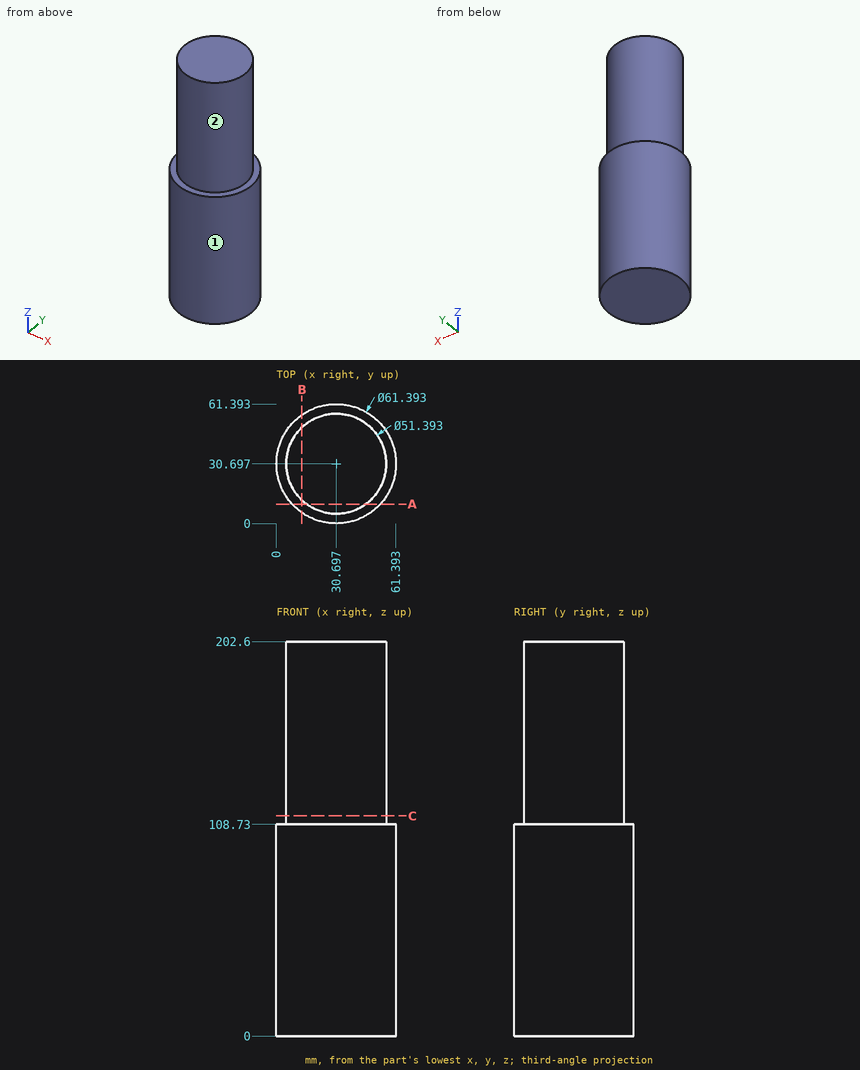
Could you check a few things on this drawing? It's one solid part, dimensions in mm from its lowest x, y, z. A direction names the side the tool comes from. Coordinates: 2 decimals unless noted, no trailing zeros. Loops run counter-clockwise (first coordinate to the right, second up) from the corner with the lowest first, then second, coordinate; pieces in that order, holes last. Notation, with made-up numbers: (28, -2) - (87, -2) arc R14 ccw to (87, 17) - close; hole circle Ø11 at (24.5, 18). An arc over 180 degrees is marked (long way). Answer as a JSON object with one key per item and string values. Group by question number.
Item 1: On a 3-axis mill with a long thin cutter (end or side, diameter ignored), from which of +Z, -Z, +X, -X, +Y, -Y can I reach the whole of each face in a straight line? I mean the marked faces 1 and 2. Say none if no direction works.
Item 2: If we section it at A-A (y = 10): List the corners of the cut face in (x, z) for me, plus the area to 3 significant figures.
Item 3: For pin 1 (1.5 mm diameter, centred on y = 27.5, z = 157.5, fed in from +X); pin 2 (5 mm diameter, centred on x = 29, z = 58, fed in from -Y); pin 3 (10 mm diameter, centred on x = 7, z = 135.5, fed in from -Y), each with a flat end and sliding along its axis, tell me the tip position at first contact or that it passes through.
Item 4: If I drill on L1, parallel to Z at x = 14, y = 55; L2, parallel to X at y = 29.5, z = 129 (1 decimal), over which ranges is the centre line in solid material (lowest first)? Write a range as from..to.
Item 5: If we section it at B-B (x = 13): List the corners of the cut face in (y, z) for me (1 decimal).
Item 6: If we section it at C-C (z = 113): List the corners of the cut face in (x, y) for me, plus the area to 3 significant figures.
Returned:
{
 "1": {"face 1": "+Z, -Z", "face 2": "+Z"},
 "2": {"outline": "(8.03, 0) - (53.37, 0) - (53.37, 108.73) - (45.93, 108.73) - (45.93, 202.6) - (15.47, 202.6) - (15.47, 108.73) - (8.03, 108.73) - close", "area": "7,790 mm²"},
 "3": {"pin 1": "stops at x = 56.28", "pin 2": "stops at y = 0", "pin 3": "stops at y = 13.07"},
 "4": {"L1": "z = 0..108.73", "L2": "x = 5..56.4"},
 "5": {"outline": "(5.6, 0) - (55.8, 0) - (55.8, 108.7) - (49.3, 108.7) - (49.3, 202.6) - (12.1, 202.6) - (12.1, 108.7) - (5.6, 108.7) - close"},
 "6": {"outline": "circle Ø51.39 at (30.7, 30.7)", "area": "2,070 mm²"}
}
